from build123d import *

# Parameters (mm, degrees)
SKETCH1_R           = 6.9
SKETCH1_R_2         = 10.9
BOSS_EXTRUDE1_DEPTH = 7
BOSS_EXTRUDE2_DEPTH = 12
CUT_EXTRUDE1_DEPTH  = 13
BOSS_EXTRUDE3_DEPTH = 26
SKETCH5_R           = 7.973914392
SKETCH5_R_2         = 4
BOSS_EXTRUDE4_DEPTH = 1.5
BOSS_EXTRUDE5_START = -1.5
SKETCH6_R           = 8.491099949
SKETCH6_R_2         = 4
BOSS_EXTRUDE5_DEPTH = 1.5
SKETCH7_R           = 2.25
CUT_EXTRUDE2_DEPTH  = 99.438905233
SCALE1_SCALE        = 1.5


with BuildPart() as part:
    # Sketch1 → Boss-Extrude1 (new body)
    with BuildSketch(Plane.XY):
        with BuildLine():
            ThreePointArc((-109.99286225, 64.498694041), (-120.238224228, 58.705152002), (-124.296770504, 47.657040238))
            Line((-124.296770504, 47.657040238), (-117.277493754, 25.812066819))
            ThreePointArc((-117.277493754, 25.812066819), (-114.348561566, 18.740999007), (-107.277493754, 15.812066819))
            add(Edge.make_bspline(
                [(-80.055270229, 25.812066819), (-90.16574855, 12.494826539), (-107.277493754, 15.812066819)],
                knots=[0, 0, 0, 1, 1, 1], degree=2))
            Line((-80.055270229, 25.812066819), (-80.055270229, 84.34418562))
            ThreePointArc((-80.055270229, 84.34418562), (-81.43033647, 86.24404293), (-83.664728026, 85.531470589))
            add(Edge.make_bspline(
                [(-109.99286225, 64.498694041), (-95.736844246, 69.471166394), (-91.130917767, 75.410465429), (-83.664728026, 85.531470589)],
                knots=[0, 0, 0, 0, 0.858728352, 0.858728352, 0.858728352, 0.858728352], degree=3))
        make_face()
        with Locations((-107.277493754, 25.812066819)):
            Circle(SKETCH1_R, mode=Mode.SUBTRACT)
        with Locations((-107.22999807, 47.657040238)):
            Circle(SKETCH1_R_2, mode=Mode.SUBTRACT)
    boss_extrude1 = extrude(amount=BOSS_EXTRUDE1_DEPTH)

    # Sketch2 → Boss-Extrude2 (add)
    with BuildSketch(Plane.XY.offset(7)):
        with BuildLine():
            Line((-85.055270217, 83.653678118), (-85.055270217, 20.583275514))
            add(Edge.make_bspline(
                [(-85.055270217, 20.583275514), (-82.371539661, 22.76114127), (-80.055270217, 25.812066834)],
                knots=[0, 0, 0, 1, 1, 1], degree=2))
            Line((-80.055270217, 25.812066834), (-80.055270229, 84.34418562))
            ThreePointArc((-80.055270229, 84.34418562), (-81.43033647, 86.24404293), (-83.664728026, 85.531470589))
            add(Edge.make_bspline(
                [(-83.664728026, 85.531470589), (-84.138702239, 84.888961408), (-84.601149423, 84.263304749), (-85.055270217, 83.653678118)],
                knots=[0, 0, 0, 0, 0.054514432, 0.054514432, 0.054514432, 0.054514432], degree=3))
        make_face()
    extrude(amount=BOSS_EXTRUDE2_DEPTH)

    # Mirror1: Boss-Extrude1 across plane
    add(boss_extrude1.mirror(Plane.XY.offset(13)))

    # Sketch3 → Cut-Extrude1 (cut)
    with BuildSketch(Plane(origin=(0, 0, 0), x_dir=(-1, 0, 0), z_dir=(0, 0, -1))):
        with BuildLine():
            Line((92.850529653, 74.397721592), (144.531216933, 88.865819457))
            Line((144.531216933, 88.865819457), (118.546118501, 29.760204905))
            add(Edge.make_bspline(
                [(107.22999807, 36.757040238), (116.864311021, 38.600442381), (118.546118501, 29.760204905)],
                knots=[0, 0, 0, 1, 1, 1], degree=2))
            ThreePointArc((107.22999807, 36.757040238), (99.522534155, 39.949576323), (96.32999807, 47.657040238))
            add(Edge.make_bspline(
                [(92.850529653, 74.397721592), (90.423550402, 60.160750292), (96.32999807, 47.657040238)],
                knots=[0, 0, 0, 1, 1, 1], degree=2))
        make_face()
    extrude(amount=-CUT_EXTRUDE1_DEPTH, mode=Mode.SUBTRACT)

    # Sketch4 → Boss-Extrude3 (add)
    with BuildSketch(Plane(origin=(0, 0, 0), x_dir=(-1, 0, 0), z_dir=(0, 0, -1))):
        with BuildLine():
            Line((83.132797407, 86.34418562), (85.055270217, 83.653678118))
            Line((85.055270217, 83.653678118), (85.055270214, 20.587782524))
            add(Edge.make_bspline(
                [(78.82999807, 27.533016311), (81.645897876, 23.355716893), (85.055270214, 20.587782524)],
                knots=[0, 0, 0, 1, 1, 1], degree=2))
            Line((78.82999807, 27.533016311), (78.82999807, 84.770259389))
            ThreePointArc((78.82999807, 84.770259389), (80.746261593, 86.200037671), (83.132797407, 86.34418562))
        make_face()
    extrude(amount=-BOSS_EXTRUDE3_DEPTH)

    # Sketch5 → Boss-Extrude4 (add)
    with BuildSketch(Plane.XY.offset(7)):
        with Locations((-107.277493754, 25.812066819)):
            Circle(SKETCH5_R)
        with Locations((-107.277493754, 25.812066819)):
            Circle(SKETCH5_R_2, mode=Mode.SUBTRACT)
    extrude(amount=-BOSS_EXTRUDE4_DEPTH)

    # Sketch6 → Boss-Extrude5 (add)
    with BuildSketch(Plane(origin=(0, 0, 19), x_dir=(-1, 0, 0), z_dir=(0, 0, -1)).offset(BOSS_EXTRUDE5_START)):
        with Locations((107.277493754, 25.812066819)):
            Circle(SKETCH6_R)
        with Locations(Location((107.277493754, 25.812066819, 0), (0, 0, 180))):
            Circle(SKETCH6_R_2, mode=Mode.SUBTRACT)
    extrude(amount=BOSS_EXTRUDE5_DEPTH)

    # Sketch7 → Cut-Extrude2 (cut, through all)
    with BuildSketch(Plane.ZY.offset(85.055270217)):
        with Locations(Location((13, 32.653678118, 0), (0, 0, 270))):
            Circle(SKETCH7_R)
        with Locations(Location((13, 52.653678118, 0), (0, 0, 270))):
            Circle(SKETCH7_R)
        with Locations(Location((13, 72.653678118, 0), (0, 0, 270))):
            Circle(SKETCH7_R)
    extrude(amount=-CUT_EXTRUDE2_DEPTH, mode=Mode.SUBTRACT)


with BuildPart() as part_1:
    # Scale1: scaled about (-91.847810328, 47.075825155, 14.137877649)
    add(part.part.scale(SCALE1_SCALE).moved(Location((45.923905164, -23.537912577, -7.068938824))))


solid = part_1.part
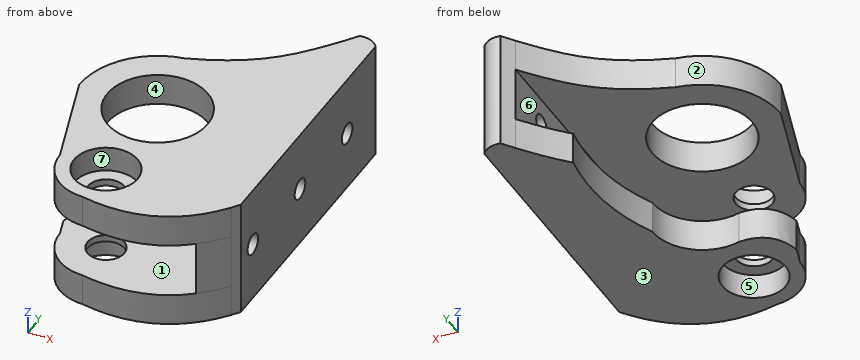
CAD build for the part. Positions are in the model's coordinates, mm. Face numbers are marked on the shaded views. A direction names the side the tool comes from. Round coordinates to 2 decimals unless told otherwise and drop trailing zeros. Loops run counter-clockwise (first coordinate to the right, second up) from the corner with the lowest first, then second, coordinate; pieces in that order, holes last. Notation, with made-up numbers: M 87.5,42 L 139.5,42 A30 ccw 139.5,74 Z; hole C 88,83.5 d2. An arc over 180 degrees is marked long. One line per question, with ' | ' between items. Start each with the question number.
Item 1: Pin check, flat tips, straight feed: pin 1 Ø2 at (y, z) = (14, -2.5) entering from +X; pin 2 Ø10 at (y, z) = (81, 6.5) entering from -X; pin 3 Ø10.5 at (x, y) = (-114, 13.5) entering from -Z. Stop position of each tip, or through.
Item 2: Wall check: line 1 (Z direction, x = -89, y = 56.5); line 2 (X direction, y = 33, z = 14.5); line 3 (X direction, y = 48.5, z = 27.5). Give the ranges that are in metal, low to high.
Item 3: Two-plate mould, pull along Z, no slides. Class the marked faces 1, 2 and 3: pulls with the +Z half, pulls with the -Z half, needs draft (parallel to the pull), parting line crosses it, or undercut.
Item 4: Cut at A-A, the plane y = 40. Write the cut outline in (x, z).
Item 5: Cut at B-B, the plane z = 14.5. State how many separate pieces and enclosed holes the cut face has, plus the area to 3 significant figures.
Item 6: Which spindle directions (+Z, -Z, +X, -X, +Y, -Y) get a long thin tool onto all of the face, cutting with end or side? Do the marked faces 4, 5, 6 and 7. Say none if no direction does.
Responses:
1) pin 1: stops at x = -74.3 | pin 2: stops at x = -92.89 | pin 3: stops at z = 1.18
2) line 1: z = -7.07 to 3.43, 21.43 to 31.93 | line 2: x = -81.66 to -72.32 | line 3: x = -140.52 to -131.26, -98.58 to -72.32
3) face 1: undercut | face 2: needs draft | face 3: pulls with the -Z half
4) outline: M -137.97,21.43 L -129.21,21.43 L -129.21,31.93 L -137.97,31.93 Z; M -100.63,-7.07 L -72.32,-7.07 L -72.32,31.93 L -100.63,31.93 L -100.63,21.43 L -81.66,21.43 L -81.66,3.43 L -100.63,3.43 Z
5) separate pieces: 4 | enclosed holes: 0 | area: 719 mm²
6) face 4: +Z, -Z | face 5: -Z | face 6: -X, +Y, -Y | face 7: +Z
